Autodesk Inventor part; units mm, degrees
ref_plane "YZ Plane" through (0, 0, 0) normal (1, 0, 0) x (0, 1, 0)
ref_plane "XZ Plane" through (0, 0, 0) normal (0, 1, 0) x (-1, 0, 0)
ref_plane "XY Plane" through (0, 0, 0) normal (0, 0, 1) x (1, 0, 0)
sketch "草图1" plane through (0, 0, 0) normal (0, 0, 1) x (1, 0, 0)
  circle A0 centre (0, 0) radius 24
  line L0 (-20.7846, -12) -> (-34.9297, 12.5)
  line L1 (-34.9297, 12.5) -> (-34.9297, 32.5)
  line L2 (-34.9297, 32.5) -> (34.9297, 32.5)
  line L3 (34.9297, 32.5) -> (34.9297, 12.5)
  line L4 (34.9297, 12.5) -> (20.7846, -12)
  line L5 (0, 0) -> (0, 15.9109)
  dimension "d0" = 48
  dimension "d1" = 15.9109
  dimension "d2" = 12.5
  dimension "d3" = 20
  dimension "d4" = 150
extrude "拉伸1" add sketch "草图1" along normal blind 5
sketch "草图2" plane through (0, 0, 5) normal (0, 0, 1) x (1, 0, 0)
  circle A0 centre (0, 0) radius 16
  circle A1 centre (0, 0) radius 12.5
  dimension "d7" = 32
  dimension "d8" = 25
extrude "拉伸2" add sketch "草图2" along normal blind 4
sketch "草图3" plane through (0, 0, 9) normal (0, 0, 1) x (1, 0, 0)
  circle A0 centre (0, 0) radius 16
  circle A1 centre (0, 0) radius 15
  dimension "d11" = 32
  dimension "d12" = 30
extrude "拉伸3" cut sketch "草图3" against normal blind 1
sketch "草图4" plane through (0, 0, 5) normal (0, 0, 1) x (1, 0, 0)
  circle A0 centre (0, 0) radius 8
  dimension "d15" = 16
extrude "拉伸4" cut sketch "草图4" against normal through all
sketch "草图5" plane through (0, 0, 5) normal (0, 0, 1) x (1, 0, 0)
  circle A0 centre (17.3205, -10) radius 1.5
  circle A1 centre (-17.3205, -10) radius 1.5
  circle A2 centre (24.9297, 22.5) radius 1.5
  circle A3 centre (-24.9297, 22.5) radius 1.5
  line L0 (-34.9297, 32.5) -> (-34.9297, 12.5)
  line L1 (34.9297, 32.5) -> (-34.9297, 32.5)
  line L2 (34.9297, 12.5) -> (34.9297, 32.5)
  arc A4 (-17.3205, -10) -> (17.3205, -10) centre (0, 0) ccw
  dimension "d18" = 3
  dimension "d19" = 3
  dimension "d20" = 3
  dimension "d21" = 3
  dimension "d22" = 10
  dimension "d23" = 10
  dimension "d24" = 10
  dimension "d25" = 10
  dimension "d26" = 10
  dimension "d27" = 20
  dimension "d28" = 10
extrude "拉伸5" cut sketch "草图5" against normal through all
sketch "草图6" plane through (0, 0, 0) normal (0, 0, -1) x (-1, 0, 0)
  circle A0 centre (17.3205, -10) radius 2.5
  circle A1 centre (-17.3205, -10) radius 2.5
  circle A2 centre (24.9297, 22.5) radius 2.5
  circle A3 centre (-24.9297, 22.5) radius 2.5
  circle A4 centre (17.3205, -10) radius 1.5
  circle A5 centre (-17.3205, -10) radius 1.5
  circle A6 centre (-24.9297, 22.5) radius 1.5
  circle A7 centre (24.9297, 22.5) radius 1.5
  point P0 (0, 0)
  dimension "d31" = 5
  dimension "d32" = 5
  dimension "d33" = 5
  dimension "d34" = 5
extrude "拉伸6" cut sketch "草图6" against normal blind 2.5
properties part number "砂轮轴端盖"
Geometry: final body of the model. Coordinates: model frame, mm. A direction names the side the tool comes from. Coordinates: 2 decimals unless noted, no trailing zeros. Loops run counter-clockwise (first coordinate to the right, second up) from the corner with the lowest first, then second, coordinate; pieces in that order, holes last. Notation, with made-up numbers: M 7,61 L 17,61 A31 ccw 17,87 Z; hole C 46,-5.5 d3. An arc over 180 degrees is marked long. Put each result on its own line as item: value.
(1) Cut plane B-B on y = 5. Return the cut outline in (x, z) (3 decimals).
Answer sheet:
outline: M -30.6,0 L -6.245,0 L -6.245,5 L -11.456,5 L -11.456,9 L -14.142,9 L -14.142,8 L -15.199,8 L -15.199,5 L -30.6,5 Z; M 6.245,0 L 30.6,0 L 30.6,5 L 15.199,5 L 15.199,8 L 14.142,8 L 14.142,9 L 11.456,9 L 11.456,5 L 6.245,5 Z
(2) Material intervals for probe 1 along Z at (x, y) = (-16.5, -2); probe 2 along Y at (x, z) = (-4, 8.5); probe 3 along Z at (x, y) = (12.5, -8.5), sorted ascending.
Answer sheet:
probe 1: z = 0 to 5
probe 2: y = -14.46 to -11.84, 11.84 to 14.46
probe 3: z = 0 to 8
(3) Draft query along Y for faces 1 (the face through (0, 17, 5)), 2 (the face through (-26, 21, 2.5)), 3 (the face through (-14.985, 0.66, 8.507)). Return one class per face: pulls with the +Y half, pulls with the -Y half, needs draft (parallel to the pull), parting line crosses it, or undercut.
Answer sheet:
face 1: needs draft
face 2: undercut
face 3: parting line crosses it
(4) First-contact query: pin 1 (14.5 mm diameter, centred on x = 0, y = 0, fed in from +Z); pin 2 (4 mm diameter, centred on x = 17.32, y = -10, fed in from +Z); pin 3 (4 mm diameter, centred on x = -7, z = 6, fed in from -Y); pin 4 (2 mm diameter, centred on y = 3.5, z = 3.5, fed in from +X). Flat tips, straight axial feed; report the tip coordinate or a pass-through.
Answer sheet:
pin 1: passes through
pin 2: stops at z = 5
pin 3: stops at y = -23.41
pin 4: stops at x = 30.31
(5) Cut plane A-A on y = 22.5. Return the cut outline in (x, z).
Answer sheet:
outline: M -34.93,0 L -27.43,0 L -27.43,2.5 L -26.43,2.5 L -26.43,5 L -34.93,5 Z; M -23.43,2.5 L -22.43,2.5 L -22.43,0 L 22.43,0 L 22.43,2.5 L 23.43,2.5 L 23.43,5 L -23.43,5 Z; M 26.43,2.5 L 27.43,2.5 L 27.43,0 L 34.93,0 L 34.93,5 L 26.43,5 Z
(6) Access query for faces 4 (the face through (0, -24, 2)), 5 (the face through (16.17, -12.22, 1.23)), 6 (the face through (-3.47, 15.62, 6.48)). Directions: +Z, -Z, +X, -X, +Y, -Y. A direction counts if a zero-diameter tool reaches every point of the face in a straight line with its end or side. Return the directions, or none.
Answer sheet:
face 4: +Z, -Z, -Y
face 5: -Z
face 6: +Z
(7) Cut plane C-C on x = -25.5. Return the cut outline in (y, z).
Answer sheet:
outline: M -3.83,0 L 20.07,0 L 20.07,2.5 L 21.11,2.5 L 21.11,5 L -3.83,5 Z; M 23.89,2.5 L 24.93,2.5 L 24.93,0 L 32.5,0 L 32.5,5 L 23.89,5 Z
(8) Cut plane D-D on z = 7.25. Return the cut outline in (x, y).
Answer sheet:
outline: C 0,0 d32; hole C 0,0 d25
